Design review of the part built by this model. Coordinates are the model's own, in mm. A direction names the side the tool comes from. Give positions to 0.01 mm unless a question says otherwise; leave off trailing zeros. Write each loop counter-clockwise with the first axis right and the second up, starting at its lowest first coordinate (ties: lowest second). Pieces come first, ordered by that corner, then holes. Notation, with made-up numbers: (-33, -21.5) - (17, -21.5) arc R11 ccw to (17, -15.5) - close; hole circle Ø10 at (-20, -15.5). An arc over 180 degrees is marked (long way). Use a Markdown table: item, result. Add a question column.
```python
from build123d import *

# Parameters (mm, degrees)
EXTRUDE_1_DEPTH      = 10
EXTRUDE_2_DEPTH      = 380
CUT_EXTRUDE_1_DEPTH  = 10
EXTRUDE_3_DEPTH      = 85
EXTRUDE_3_DEPTH_BACK = 85
SKETCH_5_R           = 5


with BuildPart() as part:
    # Sketch 1 → Extrude 1 (new body)
    with BuildSketch(Plane(origin=(0, 0, 0), x_dir=(1, 0, 0), z_dir=(0, 1, 0))):
        Polygon((0, 0), (360, 0), (180, 311.769145), align=None)
    extrude(amount=EXTRUDE_1_DEPTH)

    # Sketch 2 → Extrude 2 (add)
    with BuildSketch(Plane(origin=(0, 10, 0), x_dir=(1, 0, 0), z_dir=(0, 1, 0))):
        Polygon((360, 0), (355, 8.660254), (350, 0), align=None)
        Polygon((0, 0), (5, 8.660254), (10, 0), align=None)
        Polygon((180, 311.769145), (175, 303.108891), (185, 303.108891), align=None)
    extrude(amount=EXTRUDE_2_DEPTH)

    # Sketch 4 → Cut-Extrude 1 (cut)
    with BuildSketch(Plane(origin=(0, 0, 0), x_dir=(-1, 0, 0), z_dir=(0, -1, 0))):
        Polygon((-180, 291.769145), (-342.679492, 10), (-17.320508, 10), align=None)
    extrude(amount=-CUT_EXTRUDE_1_DEPTH, mode=Mode.SUBTRACT)

    # Sketch 5 → Extrude 3 (add, two sides: drawn at the far end of the back side and taken through both)
    with BuildSketch(Plane.ZY.offset(-180).offset(-EXTRUDE_3_DEPTH_BACK)):
        with Locations(Location((-156, 5, 0), (0, 0, 90))):
            Circle(SKETCH_5_R)
    extrude(amount=EXTRUDE_3_DEPTH + EXTRUDE_3_DEPTH_BACK)


solid = part.part
```
(1) Mouldability with a two-part tool opening along Z and no side actions: class faces 1 (the face through (180, 197, -303.109)), 2 (the face through (140.258, 4.93, -222.934)), 3 (the face through (179, 10, -6)), 4 (the face through (218.644, 4.93, -224.835)) as +Z half, -Z half, draft (parallel to the pull), parting line (faces both ways), or undercut.
(2) Insertion check: pin 1 (8 mm diameter, centred on x = 252, y = 6.5, fed in from -Z); pin 2 (3 mm diameter, centred on x = 181, y = 265.5, fed in from +Z). Each pin has a flat end and moves straight along its axis. Give the tip position at first contact, or say it passes through.
(3) Add section A-A (y = 54.5). State the section outline as (x, z) points.
(4) Add section B-B (z = -241). State the section outline as (x, y) points, and give its area (3 significant figures).
(5) Tool access review of faces 5 (the face through (99, 0, -157)), 6 (the face through (182, 5, -10)), 7 (the face through (181.104, 4.349, -160.957)): name each direction out of +Z, -Z, +X, -X, +Y, -Y from which nothing blocks a thin tool from reaching the whole face with its end or side.
(6) Add section C-C (x = 155.5). State the section outline as (y, z) points, and give its area (3 significant figures).
(7) For line 1 along Y through (x, z) = (60, -86.5); line 2 along Z through (x, y) = (180.5, 53.5); line 3 along Y through (x, z) = (106, -152.5), list the stretches that pass through material, from the lowest coordinate up.
Answers follow:
| question | item | result |
|---|---|---|
| 1 | face 1 | +Z half |
| 1 | face 2 | undercut |
| 1 | face 3 | draft |
| 1 | face 4 | undercut |
| 2 | pin 1 | z = -193.99 |
| 2 | pin 2 | z = -303.11 |
| 3 | outline | (0, 0) - (5, -8.66) - (10, 0) - close; (175, -303.11) - (180, -311.77) - (185, -303.11) - close; (350, 0) - (355, -8.66) - (360, 0) - close |
| 4 | outline | (139.14, 0) - (150.69, 0) - (150.69, 10) - (139.14, 10) - close; (209.31, 0) - (220.86, 0) - (220.86, 10) - (209.31, 10) - close |
| 4 | area | 231 mm^2 |
| 5 | face 5 | +Z, -Z, +X, -X, -Y |
| 5 | face 6 | +Y, -Y |
| 5 | face 7 | none |
| 6 | outline | (0, -269.33) - (10, -269.33) - (10, -249.33) - (0, -249.33) - close; circle Ø10 at (5, -156); (0, -10) - (10, -10) - (10, 0) - (0, 0) - close |
| 6 | area | 379 mm^2 |
| 7 | line 1 | 0 to 10 |
| 7 | line 2 | -310.9 to -303.11 |
| 7 | line 3 | 1.43 to 8.57 |
